```python
from build123d import *

# Parameters (mm, degrees)
PAD_DEPTH    = 12.7
SKETCH001_R  = 2.182812
POCKET_DEPTH = 42.7746
CHAMFER_SIZE = 1


with BuildPart() as part:
    # Sketch → Pad (new body)
    with BuildSketch(Plane.XY):
        Polygon((0, -42.7736), (22.86, -42.7736), (22.86, -37.6936), (5.08, -37.6936), (5.08, 5.08), (-12.7, 5.08), (-12.7, 0), (0, 0), align=None)
    extrude(amount=PAD_DEPTH)

    # Sketch001 → Pocket (cut, through all)
    with BuildSketch(Plane.XZ):
        with Locations((13.97, 6.35)):
            Circle(SKETCH001_R)
    extrude(amount=POCKET_DEPTH, mode=Mode.SUBTRACT)

    # Chamfer
    chamfer_edges = [part.edges().sort_by_distance(p)[0] for p in [
        (22.86, -40.2336, 0),
        (22.86, -40.2336, 12.7),
        (-12.7, 2.54, 0),
        (-12.7, 2.54, 12.7),
    ]]
    chamfer(chamfer_edges, length=CHAMFER_SIZE)


solid = part.part
```
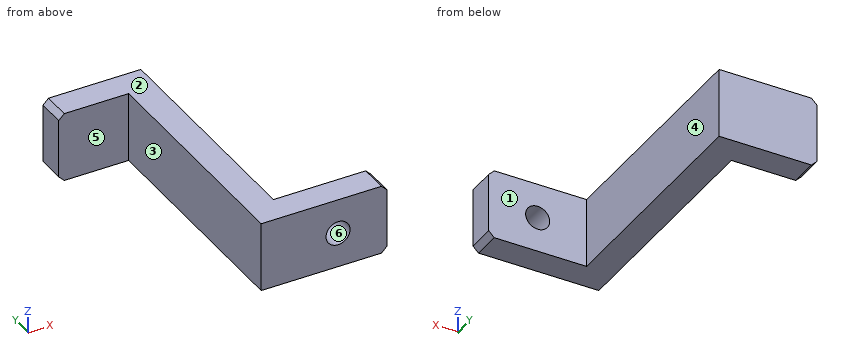
CAD build for the part. Positions are in the model's coordinates, mm. Face numbers are marked on the shaded views. A direction names the side the tool comes from. Round coordinates to 2 decimals unless told otherwise and drop trailing zeros. Loops run counter-clockwise (first coordinate to the right, second up) from the corner with the lowest first, then second, coordinate; pieces in that order, holes last. Notation, with made-up numbers: M -33.5,64 L 19.5,64 A18 cw 19.5,91 Z; hole C -26.5,63.25 d10. An arc over 180 degrees is marked long. Return JSON: item names as keys, results as strings. Group by question number.
(1) Wall check: probe 1 along Z at (x, y) = (13.97, -41.2); probe 2 along X at (y, z) = (-40.75, 6.35); probe 3 along Y at (x, z) = (-11, 9.75). Give the ranges that are in metal, low to high. Write a range as [from, to].
(2) Tool access for the marked faces 1 and 2: list every direction of +Z, -Z, +X, -X, +Y, -Y with a clear straight run to the whole face (end or side of a thin tool).
(3) Saw through at D-D, the plane y = -16.5. List the corners of the cut face in (x, z).
(4) Mould opens along X. For the marked faces 3, 4, 5 and 6 say: +X half, -X half, draft (parallel to the pull), parting line (faces both ways), or undercut.
(5) Saw through at B-B, the plane x = 13.97. List the corners of the cut face in (y, z).
(6) Saw through at C-C, the plane z = 9.5. List the corners of the cut face in (x, y), and give its area (3 significant figures).
(7) Drop flat-ended pins along their axis: P1, Ø7, axis at x = 13.97, z = 6.35, coming from the +Y side; P2, Ø6, axis at y = -32.5, z = 4.5, coming from the -X side; P3, Ø4, axis at y = -6, z = 6, coming from the +X side; P4, Ø2, axis at y = -37, z = 8, coming from the +X side. Give the stop position or say it passes through.
(8) Saw through at A-A, the plane z = 6.35. List the corners of the cut face in (x, y), and give its area (3 significant figures).
Answer list:
{
 "1": {"probe 1": "[0, 4.17], [8.53, 12.7]", "probe 2": "[0, 11.79], [16.15, 22.86]", "probe 3": "[0, 5.08]"},
 "2": {"face 1": "+Z, -Z, +X, +Y", "face 2": "+Z, +X, -X, +Y, -Y"},
 "3": {"outline": "M 0,0 L 5.08,0 L 5.08,12.7 L 0,12.7 Z"},
 "4": {"face 3": "-X half", "face 4": "+X half", "face 5": "draft", "face 6": "undercut"},
 "5": {"outline": "M -42.77,0 L -37.69,0 L -37.69,4.17 L -42.77,4.17 Z; M -42.77,8.53 L -37.69,8.53 L -37.69,12.7 L -42.77,12.7 Z"},
 "6": {"outline": "M -12.7,0 L 0,0 L 0,-42.77 L 22.86,-42.77 L 22.86,-37.69 L 5.08,-37.69 L 5.08,5.08 L -12.7,5.08 Z", "area": "398 mm2"},
 "7": {"P1": "y = -37.69", "P2": "x = 0", "P3": "x = 5.08", "P4": "x = 22.86"},
 "8": {"outline": "M -12.7,0 L 0,0 L 0,-42.77 L 11.79,-42.77 L 11.79,-37.69 L 5.08,-37.69 L 5.08,5.08 L -12.7,5.08 Z; M 16.15,-42.77 L 22.86,-42.77 L 22.86,-37.69 L 16.15,-37.69 Z", "area": "376 mm2"}
}
